```python
from build123d import *

# Parameters (mm, degrees)
SKETCH1_W             = 680
SKETCH1_H             = 340
SKETCH1_R             = 11.5
SKETCH1_R_2           = 20
BOSS_EXTRUDE1_DEPTH   = 10
CHAMFER1_SIZE         = 2
M4X0_7_TAPPED_HOLE1_D = 3.3
MIRROR2_COPY_1_D      = 3.3
M4X0_7_TAPPED_HOLE2_D = 3.3
LPATTERN1_COUNT       = 3
LPATTERN1_PITCH       = 105
LPATTERN1_COL_COUNT   = 3
LPATTERN1_COL_PITCH   = 105


with BuildPart() as part:
    # Sketch1 → Boss-Extrude1 (new body)
    with BuildSketch(Plane(origin=(0, 0, 0), x_dir=(1, 0, 0), z_dir=(0, 1, 0))):
        Rectangle(SKETCH1_W, SKETCH1_H)
        with Locations(Location((-320, -150, 0), (0, 0, 270))):
            Circle(SKETCH1_R, mode=Mode.SUBTRACT)
        with Locations(Location((0, 0, 0), (0, 0, 270))):
            Circle(SKETCH1_R_2, mode=Mode.SUBTRACT)
        with Locations(Location((-320, 150, 0), (0, 0, 90))):
            Circle(SKETCH1_R, mode=Mode.SUBTRACT)
        with Locations(Location((320, 150, 0), (0, 0, 270))):
            Circle(SKETCH1_R, mode=Mode.SUBTRACT)
        with Locations(Location((320, -150, 0), (0, 0, 90))):
            Circle(SKETCH1_R, mode=Mode.SUBTRACT)
        with Locations(Location((-105, 0, 0), (0, 0, 270))):
            Circle(SKETCH1_R_2, mode=Mode.SUBTRACT)
        with Locations(Location((-210, 0, 0), (0, 0, 270))):
            Circle(SKETCH1_R_2, mode=Mode.SUBTRACT)
        with Locations(Location((105, 0, 0), (0, 0, 90))):
            Circle(SKETCH1_R_2, mode=Mode.SUBTRACT)
        with Locations(Location((210, 0, 0), (0, 0, 90))):
            Circle(SKETCH1_R_2, mode=Mode.SUBTRACT)
    extrude(amount=BOSS_EXTRUDE1_DEPTH)

    # Chamfer1
    chamfer1_edges = [part.edges().sort_by_distance(p)[0] for p in [
        (-340, 5, -170),
        (340, 5, -170),
        (340, 5, 170),
        (-340, 5, 170),
    ]]
    chamfer(chamfer1_edges, length=CHAMFER1_SIZE)

    # M4x0.7 Tapped Hole1 (through all)
    with Locations(Plane(origin=(-331.313708499, 10, 138.686291501), x_dir=(0, 0, 1), z_dir=(0, 1, 0))):
        with Locations((0, 0), (0, 22.627416998), (22.627416998, 22.627416998), (22.627416998, 0)):
            m4x0_7_tapped_hole1 = Hole(M4X0_7_TAPPED_HOLE1_D / 2)

    # Mirror1: M4x0.7 Tapped Hole1 across plane
    add(m4x0_7_tapped_hole1.mirror(Plane.XY), mode=Mode.SUBTRACT)

    # Mirror2: M4x0.7 Tapped Hole1 across plane
    add(m4x0_7_tapped_hole1.mirror(Plane(origin=(0, 0, 0), x_dir=(0, 0, 1), z_dir=(1, 0, 0))), mode=Mode.SUBTRACT)

    # Mirror2 copy 1 (through all)
    with Locations(Plane(origin=(331.313708499, 10, -138.686291501), x_dir=(0, 0, -1), z_dir=(0, 1, 0))):
        with Locations((0, 0), (0, 22.627416998), (22.627416998, 22.627416998), (22.627416998, 0)):
            Hole(MIRROR2_COPY_1_D / 2)

    # M4x0.7 Tapped Hole2 (through all)
    with Locations(Plane(origin=(-22.083647797, 10, -12.75), x_dir=(0, 0, 1), z_dir=(0, 1, 0))):
        with Locations((0, 0), (0, 44.167295594), (38.25, 22.083647797)):
            m4x0_7_tapped_hole2 = Hole(M4X0_7_TAPPED_HOLE2_D / 2)

    # LPattern1: M4x0.7 Tapped Hole2 ×3
    with Locations(*[(i * LPATTERN1_PITCH, 0, 0) for i in range(1, LPATTERN1_COUNT)]):
        add(m4x0_7_tapped_hole2, mode=Mode.SUBTRACT)

    # LPattern1 col: M4x0.7 Tapped Hole2 ×3
    with Locations(*[(-i * LPATTERN1_COL_PITCH, 0, 0) for i in range(1, LPATTERN1_COL_COUNT)]):
        add(m4x0_7_tapped_hole2, mode=Mode.SUBTRACT)


solid = part.part
```
Can you work these out from the model? Positions are in its coordinate system, mm. Coordinates: 2 decimals unless noted, no trailing zeros. Order: outer loops, then holes, each group sorted by start corner. A loop starts at its lowest first (then second) coordinate and runs counter-clockwise, first axis right, second up.
1. I'm going to push flat-ended pins straight in: pin 1 (5.5 mm diameter, centred on x = -105, z = 25.5, fed in from +Y); pin 2 (2 mm diameter, centred on x = 331.31, z = -138.69, fed in from +Y). Where does each tip first touch, or does it pass through?
2. If we section it at D-D (x = -115.5): Please give me the cut outline in (y, z), then the cut area to 3 significant figures.
3. I need wall thicknesses on line 1 (X direction, y = 2.25, z = 25.5); line 2 (X direction, y = 1.75, z = 4); line 3 (Z direction, x = -16.5, y = 1.75). Which ranges of each line are inside material? Lowest first, please.
4. If we section it at A-A (z = -150): Please give me the cut outline in (x, y).
5. If we section it at C-C (x = 320): Please give me the cut outline in (y, z).
6. If we section it at B-B (z = 0): Please give me the cut outline in (x, y), then the cut area to 3 significant figures.
7. Thinking about a two-plate mould opening in Z: for faces 1 (the face through (-5, 10, -40)), 2 (the face through (-190.17, 4.93, -2.6)), which applies, +Z half, -Z half, draft (parallel to the pull), parting line (faces both ways), or undercut?
Entries:
1. pin 1: stops at y = 10
1. pin 2: passes through
2. outline: (0, -170) - (10, -170) - (10, -17.02) - (0, -17.02) - close; (0, 17.02) - (10, 17.02) - (10, 170) - (0, 170) - close
2. area: 3,060 mm2
3. line 1: x = -340 to -211.65, -208.35 to -106.65, -103.35 to -1.65, 1.65 to 103.35, 106.65 to 208.35, 211.65 to 340
3. line 2: x = -340 to -229.6, -190.4 to -124.6, -85.4 to -19.6, 19.6 to 85.4, 124.6 to 190.4, 229.6 to 340
3. line 3: z = -170 to -11.3, 11.3 to 170
4. outline: (-340, 0) - (-331.5, 0) - (-331.5, 10) - (-340, 10) - close; (-308.5, 0) - (308.5, 0) - (308.5, 10) - (-308.5, 10) - close; (331.5, 0) - (340, 0) - (340, 10) - (331.5, 10) - close
5. outline: (0, -170) - (10, -170) - (10, -161.5) - (0, -161.5) - close; (0, -138.5) - (10, -138.5) - (10, 138.5) - (0, 138.5) - close; (0, 161.5) - (10, 161.5) - (10, 170) - (0, 170) - close
6. outline: (-340, 0) - (-230, 0) - (-230, 10) - (-340, 10) - close; (-190, 0) - (-125, 0) - (-125, 10) - (-190, 10) - close; (-85, 0) - (-20, 0) - (-20, 10) - (-85, 10) - close; (20, 0) - (85, 0) - (85, 10) - (20, 10) - close; (125, 0) - (190, 0) - (190, 10) - (125, 10) - close; (230, 0) - (340, 0) - (340, 10) - (230, 10) - close
6. area: 4,800 mm2
7. face 1: draft
7. face 2: undercut
